from build123d import *

# Parameters (mm, degrees)
SKETCH1_R               = 6.35
SKETCH1_R_2             = 7.220009846
BOSS_EXTRUDE1_DEPTH     = 38.1
SKETCH2_W               = 50.8
SKETCH2_H               = 25.4
CUT_EXTRUDE1_DEPTH      = 6.35
CUT_EXTRUDE2_DEPTH      = 131.862598214
CUT_EXTRUDE2_DEPTH_BACK = 131.862598214
SKETCH5_W               = 76.2
SKETCH5_H               = 12.7
SKETCH4_W               = 76.2
SKETCH4_H               = 6.35
CUT_EXTRUDE3_DEPTH      = 31.75
SKETCH6_R               = 7.62
SKETCH6_R_2             = 6.35
EXTRUDE_THIN1_DEPTH     = 12.7
SKETCH7_W               = 32.699691946
SKETCH7_H               = 6.35
CUT_EXTRUDE4_DEPTH      = 19.05


with BuildPart() as part:
    # Sketch1 → Boss-Extrude1 (new body)
    with BuildSketch(Plane.XY):
        with BuildLine():
            Line((-104.416317992, 20.723849372), (47.983682008, 20.723849372))
            ThreePointArc((47.983682008, 20.723849372), (67.033682008, 1.673849372), (47.983682008, -17.376150628))
            Line((47.983682008, -17.376150628), (-104.416317992, -17.376150628))
            ThreePointArc((-104.416317992, -17.376150628), (-123.466317992, 1.673849372), (-104.416317992, 20.723849372))
        make_face()
        with Locations(Location((47.983682008, 1.673849372, 0), (0, 0, 180))):
            Circle(SKETCH1_R, mode=Mode.SUBTRACT)
        with Locations(Location((-104.416317992, 1.673849372, 0), (0, 0, 180))):
            Circle(SKETCH1_R_2, mode=Mode.SUBTRACT)
    extrude(amount=BOSS_EXTRUDE1_DEPTH)

    # Sketch2 → Cut-Extrude1 (cut)
    with BuildSketch(Plane.XY):
        with Locations((-91.716317992, 1.673849372)):
            Rectangle(SKETCH2_W, SKETCH2_H)
    extrude(amount=CUT_EXTRUDE1_DEPTH, mode=Mode.SUBTRACT)

    # Sketch5 → Cut-Extrude2 (cut, two sides: drawn at the far end of the back side and taken through both)
    with BuildSketch(Plane(origin=(0, 0, 0), x_dir=(1, 0, 0), z_dir=(0, 1, 0)).offset(-CUT_EXTRUDE2_DEPTH_BACK)):
        with Locations((35.283682008, -19.05)):
            Rectangle(SKETCH5_W, SKETCH5_H)
    extrude(amount=CUT_EXTRUDE2_DEPTH + CUT_EXTRUDE2_DEPTH_BACK, mode=Mode.SUBTRACT)

    # Sketch4 → Cut-Extrude3 (cut)
    with BuildSketch(Plane(origin=(0, 20.723849372, 0), x_dir=(1, 0, 0), z_dir=(0, 1, 0))):
        with Locations((-79.016317992, -19.05)):
            Rectangle(SKETCH4_W, SKETCH4_H)
    extrude(amount=-CUT_EXTRUDE3_DEPTH, mode=Mode.SUBTRACT)

    # Sketch6 → Extrude-Thin1 (add)
    with BuildSketch(Plane(origin=(0, 0, 38.1), x_dir=(-1, 0, 0), z_dir=(0, 0, -1))):
        with Locations((104.416317992, 1.673849372)):
            Circle(SKETCH6_R)
        with Locations((104.416317992, 1.673849372)):
            Circle(SKETCH6_R_2, mode=Mode.SUBTRACT)
    extrude(amount=EXTRUDE_THIN1_DEPTH)

    # Sketch7 → Cut-Extrude4 (cut)
    with BuildSketch(Plane(origin=(0, 20.723849372, 0), x_dir=(1, 0, 0), z_dir=(0, 1, 0))):
        with Locations((-118.381657109, -19.05)):
            Rectangle(SKETCH7_W, SKETCH7_H)
    extrude(amount=-CUT_EXTRUDE4_DEPTH, mode=Mode.SUBTRACT)


solid = part.part
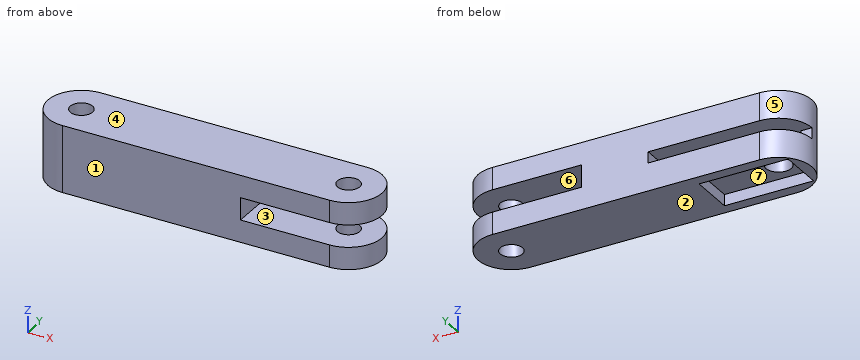
The model under review builds one solid part; all positions refer to its coordinate system, in mm. Face numbers are marked on the shaded views. A direction names the side the tool comes from. Coordinates: 2 decimals unless noted, no trailing zeros. Loops run counter-clockwise (first coordinate to the right, second up) from the corner with the lowest first, then second, coordinate; pieces in that order, holes last. Notation, with made-up numbers: M 78.5,46 L 124.5,46 A36 cw 124.5,85 Z; hole C 84.5,28 d11. An arc over 180 degrees is marked long. Put each result on its own line as item: value. Start each with the question number.
Q1. Add section D-D (z = 19). Write out the cut boundary in (x, y).
Q2. The part is to be moulded in two halves that separate along Z. For the marked faces 1, 2, 3 and 4, say which applies: +Z half, -Z half, draft (parallel to the pull), parting line (faces both ways), or undercut.
Q3. For the marked faces 5, 6 and 7, list the 3-axis set-ups (+Z, -Z, +X, -X, +Y, -Y) from which the entire face can be reached by the end or side of a thin tool; tool diameter is ignored.
Q4. Clearance check with flat-ended pins moving along their axes: pin 1 (3 mm diameter, centred on x = -84, z = 19, fed in from +Y); pin 2 (9.5 mm diameter, centred on x = -91.5, y = 12.5, fed in from -Z); pin 3 (2 mm diameter, centred on y = -13, z = 8, fed in from -X); pin 4 (1 mm diameter, centred on y = 5.5, z = 7, fed in from +X). State where each tip first meets the part, or that it passes through.
Q5. Add section C-C (x = -73). Write out the cut boundary in (y, z) (3 decimals).
Q6. Add section A-A (z = 11). Write out the cut boundary in (x, y), and give its area (3 significant figures).
Q7. Wall thickness on line 1 (Z direction, x = 23, y = 2); line 2 (X direction, y = 7, z = 28); line 3 (Z direction, x = -89, y = 17) (3 decimals): over which ranges is each line inside the solid? List them lowest first.
Q8. Add section B-B (x = 46). Write out the cut boundary in (y, z), and give its area (3 significant figures).
Answers:
1. outline: M -123.47,1.67 A19.05 ccw -104.42,-17.38 L -2.82,-17.38 L -2.82,20.72 L -40.92,20.72 L -40.92,-11.03 L -117.12,-11.03 L -117.12,1.67 Z
2. face 1: draft
2. face 2: -Z half
2. face 3: undercut
2. face 4: +Z half
3. face 5: +Z, -Z, -X
3. face 6: +X, +Y, -Y
3. face 7: -Z
4. pin 1: stops at y = -11.03
4. pin 2: stops at z = 0
4. pin 3: stops at x = -117.68
4. pin 4: stops at x = 66.74
5. outline: M -17.376,0 L -11.026,0 L -11.026,6.35 L 14.374,6.35 L 14.374,0 L 20.724,0 L 20.724,15.875 L -11.026,15.875 L -11.026,22.225 L 20.724,22.225 L 20.724,38.1 L -17.376,38.1 Z
6. outline: M -104.42,-17.38 L 47.98,-17.38 A19.05 ccw 47.98,20.72 L -104.42,20.72 A19.05 ccw Z; hole C -104.42,1.67 d14.44; hole C 47.98,1.67 d12.7
6. area: 6,660 mm^2
7. line 1: z = 0 to 12.7, 25.4 to 38.1
7. line 2: x = -122.71 to -107.87, -100.96 to 44.53, 51.44 to 66.27
7. line 3: z = 0 to 15.875, 22.225 to 38.1
8. outline: M -17.38,0 L -4.36,0 L -4.36,12.7 L -17.38,12.7 Z; M -17.38,25.4 L -4.36,25.4 L -4.36,38.1 L -17.38,38.1 Z; M 7.71,0 L 20.72,0 L 20.72,12.7 L 7.71,12.7 Z; M 7.71,25.4 L 20.72,25.4 L 20.72,38.1 L 7.71,38.1 Z
8. area: 661 mm^2
